CAD build for the part. Positions are in the model's coordinates, mm. Give positions to 0.01 mm unless a question says otherwise; leave off trailing zeros. Write each loop counter-clockwise with the first axis right and the second up, starting at its lowest first coordinate (ties: lowest second). Pieces come first, ordered by that corner, then holes. Notation, with made-up numbers: (55, 46) -> (95, 46) arc R28 ccw to (95, 84) -> close; hole circle Ø10 at (84, 63). An arc over 180 degrees is marked (long way). Answer in a Markdown table with one row per item. Add a question column.
```python
from build123d import *

# Parameters (mm, degrees)
F0_R           = 8.5
F0_R_2         = 7
F1_DEPTH       = 30
F2_R           = 20
F3_DEPTH       = 34
F5_D           = 14
F5_CSINK_D     = 40
F5_CSINK_ANGLE = 47
F6_SIZE2       = 10.919107028
F6_SIZE        = 30
F7_SIZE2       = 0.5
F7_SIZE        = 0.7140740034
F8_W           = 87.9276357591
F8_H           = 44.8519736528
F9_DEPTH       = 20.001
F10_DEPTH      = 20.001


with BuildPart() as f1:
    # F0 (on Top) → F1 (new body)
    with BuildSketch(Plane.XY):
        Circle(F0_R)
        Circle(F0_R_2, mode=Mode.SUBTRACT)
    extrude(amount=F1_DEPTH)

    # F2 (on face) → F3 (join)
    with BuildSketch(Plane(origin=(0, 0, 0), x_dir=(1, 0, 0), z_dir=(0, 0, -1))):
        Circle(F2_R)
    extrude(amount=F3_DEPTH)

    # F5 (through all)
    with Locations(Plane(origin=(0, 0, -34), x_dir=(1, 0, 0), z_dir=(0, 0, -1))):
        with Locations((0, 0)):
            CounterSinkHole(F5_D / 2, F5_CSINK_D / 2, counter_sink_angle=F5_CSINK_ANGLE)

    # F6
    f6_edges = [f1.edges().sort_by_distance(p)[0] for p in [
        (-20, 0, 0),
    ]]
    f6_side = f1.faces().sort_by_distance((-20, 0, -17))[0]
    chamfer(f6_edges, length=F6_SIZE, length2=F6_SIZE2, reference=f6_side)

    # F7
    f7_edges = [f1.edges().sort_by_distance(p)[0] for p in [
        (-9.080893, 0, 0),
    ]]
    f7_side = f1.faces().sort_by_distance((-14.540446, 0, -15))[0]
    chamfer(f7_edges, length=F7_SIZE, length2=F7_SIZE2, reference=f7_side)

    # F8 (on Front) → F9 (cut, through all)
    with BuildSketch(Plane.XZ):
        with Locations((9.7697358578, -22.4259868264)):
            Rectangle(F8_W, F8_H)
    extrude(amount=-F9_DEPTH, mode=Mode.SUBTRACT)

    # F8 (on Front) → F10 (cut, through all)
    with BuildSketch(Plane.XZ):
        with Locations((9.7697358578, -22.4259868264)):
            Rectangle(F8_W, F8_H)
    extrude(amount=F10_DEPTH, mode=Mode.SUBTRACT)


solid = f1.part
```
Item 1: Slice it at C-C, the plane z = 2. List the corners of the cut face in (x, y).
Item 2: Slice it at A-A, the plane y = 0. List the corners of the cut face in (x, z).
Item 3: Drop flat-ended pins along their axis: pin 1 Ø2 at (x, z) = (-3, 23.5) entering from +Y; pin 2 Ø1 at (x, z) = (-6.5, 5.5) entering from -Y; pin 3 Ø2 at (x, z) = (-6, 23) entering from +Y. Give the stop position or say it passes through.
Item 4: Probe L1, parallel to Y at x = 0, z = 24.25; L2, parallel to Y at x = 2.5, z = 4; L3, parallel to X at y = -2, z = 17.5. List the from-to ranges inside material, lowest first. Write a range as from..to.
Item 5: Mould opens along Y. For faces 1 (the face through (2, -7, 0)), 2 (the face through (4.57, 7.167, 14.79)), 3 (the face through (6.466, -2.681, 14.79)) say: released by +Y, released by -Y, zero draft, split by the parting line, or undercut.
Answer key:
| question | item | result |
|---|---|---|
| 1 | outline | circle Ø17 at (0, 0); hole circle Ø14 at (0, 0) |
| 2 | outline | (-8.5, 0) -> (-7, 0) -> (-7, 30) -> (-8.5, 30) -> close; (7, 0) -> (8.5, 0) -> (8.5, 30) -> (7, 30) -> close |
| 3 | pin 1 | stops at y = 8.26 |
| 3 | pin 2 | stops at y = -6.02 |
| 3 | pin 3 | stops at y = 6.87 |
| 4 | L1 | y = -8.5..-7, 7..8.5 |
| 4 | L2 | y = -8.12..-6.54, 6.54..8.12 |
| 4 | L3 | x = -8.26..-6.71, 6.71..8.26 |
| 5 | face 1 | zero draft |
| 5 | face 2 | split by the parting line |
| 5 | face 3 | undercut |
